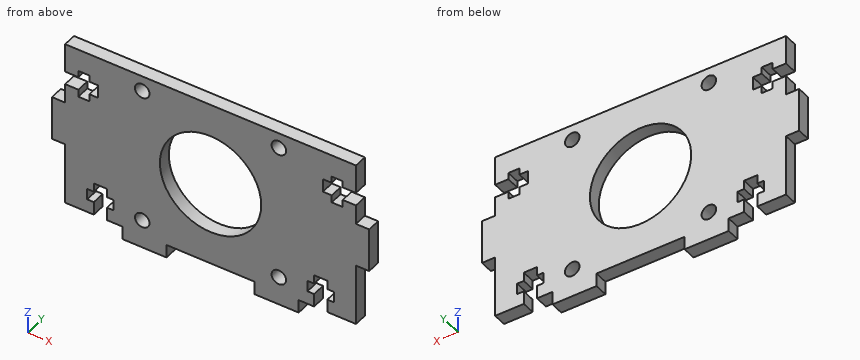
```python
from build123d import *

# Parameters (mm, degrees)
F0_R     = 1.65
F0_R_2   = 11.5
F1_DEPTH = 3
F3_DEPTH = 3


# Not quite as in the source:
# - a feature names something its author has since deleted; it is built from what else it names


with BuildPart() as f1:
    # F0 (on Front) → F1 (new body)
    with BuildSketch(Plane.XZ):
        Polygon((33, 5), (33, 19), (-33, 19), (-33, 5), (-36, 5), (-36, -5), (-33, -5), (-33, -19), (-20, -19), (-20, -22), (-10, -22), (-10, -19), (0, -19), (10, -19), (10, -22), (20, -22), (20, -19), (33, -19), (33, -5), (36, -5), (36, 5), align=None)
        with Locations((-15.5, -15.5)):
            Circle(F0_R, mode=Mode.SUBTRACT)
        with Locations((15.5, -15.5)):
            Circle(F0_R, mode=Mode.SUBTRACT)
        with Locations((-15.5, 15.5)):
            Circle(F0_R, mode=Mode.SUBTRACT)
        Circle(F0_R_2, mode=Mode.SUBTRACT)
        with Locations((15.5, 15.5)):
            Circle(F0_R, mode=Mode.SUBTRACT)
    extrude(amount=F1_DEPTH)

    # F2 (on face) → F3 (cut, through all)
    with BuildSketch(Plane.XZ.offset(3)):
        Polygon((23.5, -16), (23.5, -19), (26.5, -19), (26.5, -16), (28, -16), (28, -13.5), (26.5, -13.5), (26.5, -11.5), (23.5, -11.5), (23.5, -13.5), (22, -13.5), (22, -16), align=None)
        Polygon((-26.5, -19), (-23.5, -19), (-23.5, -16), (-22, -16), (-22, -13.5), (-23.5, -13.5), (-23.5, -11.5), (-26.5, -11.5), (-26.5, -13.5), (-28, -13.5), (-28, -16), (-26.5, -16), align=None)
        Polygon((30, 9.4201220199), (33, 9.4201220199), (33, 11), (33, 12.4201220199), (30, 12.4201220199), (30, 13.9201220199), (27.5, 13.9201220199), (27.5, 12.4201220199), (25.5, 12.4201220199), (25.5, 9.4201220199), (27.5, 9.4201220199), (27.5, 7.7319853008), (30, 7.7319853008), align=None)
        Polygon((-30, 12.4201220199), (-33, 12.4201220199), (-33, 11), (-33, 9.4201220199), (-30, 9.4201220199), (-30, 7.7319853008), (-27.5, 7.7319853008), (-27.5, 9.4201220199), (-25.5, 9.4201220199), (-25.5, 12.4201220199), (-27.5, 12.4201220199), (-27.5, 13.9201220199), (-30, 13.9201220199), align=None)
    extrude(amount=-F3_DEPTH, mode=Mode.SUBTRACT)


solid = f1.part
```
Geometry: final body of the model. Coordinates: model frame, mm. Coordinates: 2 decimals unless noted, no trailing zeros. Order: outer loops, then holes, each group sorted by start corner. A loop starts at its lowest first (then second) coordinate and runs counter-clockwise, first axis right, second up. Notation, with made-up numbers: (24.5, 66) - (58.5, 66) arc R29 ccw to (58.5, 101) - close; hole circle Ø7 at (69.25, 68.5). An arc over 180 degrees is marked (long way). Write each question's results on one line, items separated by ' | '.
(1) Line query: line 1 (Z direction, x = 15.5, y = -2.1); line 2 (X direction, y = -1.75, z = -17.5); line 3 (Z direction, x = 0, y = -2.35). Output: solid intervals per line, ascending. Write a range as [from, to].
Values found:
line 1: z = [-22, -17.15], [-13.85, 13.85], [17.15, 19] | line 2: x = [-33, -26.5], [-23.5, 23.5], [26.5, 33] | line 3: z = [-19, -11.5], [11.5, 19]
(2) First-contact query: pin 1 Ø0.9 at (y, z) = (-1.5, -20) entering from +X; pin 2 Ø1.5 at (y, z) = (-1, -17) entering from +X; pin 3 Ø0.9 at (x, y) = (-22, -2) entering from -Z. Flat tips, straight axial feed; report the tip coordinate or a pass-through.
Values found:
pin 1: stops at x = 20 | pin 2: stops at x = 33 | pin 3: stops at z = -19
(3) Section query A-A, the plane z = 15.5. Return the cut outline in (x, y).
Values found:
outline: (-33, -3) - (-17.15, -3) - (-17.15, 0) - (-33, 0) - close; (-13.85, -3) - (13.85, -3) - (13.85, 0) - (-13.85, 0) - close; (17.15, -3) - (33, -3) - (33, 0) - (17.15, 0) - close
(4) Section query D-D, the plane z = 4. Return the cut outline in (x, y), plus the area to 3 significant figures.
Values found:
outline: (-36, -3) - (-10.78, -3) - (-10.78, 0) - (-36, 0) - close; (10.78, -3) - (36, -3) - (36, 0) - (10.78, 0) - close | area: 151 mm²
(5) Section query B-B, the plane x = 5. Return the cut outline in (y, z), plus the area to 3 significant figures.
Values found:
outline: (-3, -19) - (0, -19) - (0, -10.36) - (-3, -10.36) - close; (-3, 10.36) - (0, 10.36) - (0, 19) - (-3, 19) - close | area: 51.9 mm²
(6) Section query C-C, the plane x = 15.5. Return the cut outline in (y, z), plus the area to 3 significant figures.
Values found:
outline: (-3, -22) - (0, -22) - (0, -17.15) - (-3, -17.15) - close; (-3, -13.85) - (0, -13.85) - (0, 13.85) - (-3, 13.85) - close; (-3, 17.15) - (0, 17.15) - (0, 19) - (-3, 19) - close | area: 103 mm²
